Verification items for the finished model (mm, model axes). Give positions to 0.01 mm unless a question says otherwise; leave off trailing zeros. Write each loop counter-clockwise with the first axis right and the second up, starting at its lowest first coordinate (ties: lowest second). Pieces come first, ordered by that corner, then holes. Notation, with made-up numbers: (-1.75, 80.5) - (57.25, 80.5) arc R28 cw to (57.25, 106.5) - close; hole circle Ø10 at (18.25, 68). An arc over 180 degrees is marked (long way). Put each result on its own line as item: value.
Autodesk Inventor part; units mm, degrees
ref_plane "YZ Plane" through (0, 0, 0) normal (1, 0, 0) x (0, 1, 0)
ref_plane "XZ Plane" through (0, 0, 0) normal (0, 1, 0) x (-1, 0, 0)
ref_plane "XY Plane" through (0, 0, 0) normal (0, 0, 1) x (1, 0, 0)
sketch "Sketch1" plane through (0, 0, 0) normal (0, 1, 0) x (-1, 0, 0)
  circle A0 centre (0, 0) radius 9
  dimension "d0" = 18
extrude "Extrusion1" add sketch "Sketch1" along normal blind 3.5
sketch "Sketch2" plane through (0, 3.5, 0) normal (0, 1, 0) x (1, 0, 0)
  circle A0 centre (0, 0) radius 2.75
  dimension "d3" = 5.5
extrude "Extrusion2" add sketch "Sketch2" along normal blind 10
sketch "Sketch3" plane through (0, 13.5, 0) normal (0, 1, 0) x (1, 0, 0)
  circle A0 centre (0, 0) radius 1.125
  dimension "d6" = 2.25
extrude "Extrusion3" cut sketch "Sketch3" against normal up to surface (13.5 mm away)
properties part number "Belt_Bearing_Holder"
Q1. Release check for a two-part mould opening along Z. For faces 1 (the face through (-0.146, 6.844, -1.115)), 2 (the face through (-0.596, 8.43, -2.685)), 3 (the face through (2.1, 3.5, 2.1)) record: released by +Z, released by -Z, zero draft, split by the parting line, or undercut.
Answers follow:
face 1: undercut
face 2: split by the parting line
face 3: zero draft
Q2. Section check A-A, the plane x = 0. Record the cut outline in (y, z) (3 decimals), plus the area to 3 significant figures.
Answers follow:
outline: (0, -9) - (3.5, -9) - (3.5, -2.75) - (13.5, -2.75) - (13.5, -1.125) - (0, -1.125) - close; (0, 1.125) - (13.5, 1.125) - (13.5, 2.75) - (3.5, 2.75) - (3.5, 9) - (0, 9) - close
area: 87.6 mm2
Q3. Scan lines: line 1 along Z through (x, y) = (0, 8) (3 decimals); line 2 along Y through (x, z) = (5.25, 5). Record each from-to range of solid material in increasing order.
Answers follow:
line 1: z = -2.75 to -1.125, 1.125 to 2.75
line 2: y = 0 to 3.5
Q4. Section check B-B, the plane z = 0. Record the cut outline in (x, y) (3 decimals), plus the area to 3 significant figures.
Answers follow:
outline: (-9, 0) - (-1.125, 0) - (-1.125, 13.5) - (-2.75, 13.5) - (-2.75, 3.5) - (-9, 3.5) - close; (1.125, 0) - (9, 0) - (9, 3.5) - (2.75, 3.5) - (2.75, 13.5) - (1.125, 13.5) - close
area: 87.6 mm2
Q5. Section check D-D, the plane x = -6.5. Record the cut outline in (y, z).
Answers follow:
outline: (0, -6.22) - (3.5, -6.22) - (3.5, 6.22) - (0, 6.22) - close
Q6. Go/stop test with flat-tipped pins: pin 1 Ø6 at (x, z) = (-3, 2.5) entering from -Y; pin 2 Ø5 at (x, z) = (3, -6) entering from +Y; pin 3 Ø5 at (y, z) = (2, 6) entering from +X; pin 4 Ø6 at (y, z) = (11, 5.5) entering from +X. Record where each tip stops, or that it passes through.
Answers follow:
pin 1: stops at y = 0
pin 2: stops at y = 3.5
pin 3: stops at x = 8.29
pin 4: stops at x = 1.15
Q7. Section check C-C, the plane y = 6. Record the cut outline in (x, z) (3 decimals), plus the area to 3 significant figures.
Answers follow:
outline: circle Ø5.5 at (0, 0); hole circle Ø2.25 at (0, 0)
area: 19.8 mm2
